from build123d import *

# Parameters (mm, degrees)
SKETCH1_W               = 38.1
SKETCH1_H               = 127
BOSS_EXTRUDE1_DEPTH     = 57.15
SKETCH2_W               = 21.59
SKETCH2_H               = 254
CUT_EXTRUDE1_DEPTH      = 46.99
CUT_EXTRUDE2_DEPTH      = 94.541341128
CUT_EXTRUDE2_DEPTH_BACK = 94.541341128
SKETCH3_R               = 5.08
CUT_EXTRUDE8_START      = -38.1
CUT_EXTRUDE8_DEPTH      = 38.1
SKETCH12_W              = 19.558
SKETCH12_H              = 12.7
CUT_EXTRUDE9_DEPTH      = 140.549828341
SKETCH13_R              = 2.413
CUT_EXTRUDE10_DEPTH     = 80.81826227
F_3_CLEARANCE_HOLE1_D   = 4.5
SKETCH16_R              = 2.2479
CUT_EXTRUDE11_DEPTH     = 93.011478034
CUT_EXTRUDE13_DEPTH     = 6
CUT_EXTRUDE14_DEPTH     = 93.011478034
FILLET3_R               = 2.54


# Read off the part's stored shape, not the designer's step: Cut-Extrude8
with BuildPart() as part:
    # Sketch1 → Boss-Extrude1 (new body)
    with BuildSketch(Plane(origin=(0, 0, 0), x_dir=(1, 0, 0), z_dir=(0, 1, 0))):
        Rectangle(SKETCH1_W, SKETCH1_H)
    extrude(amount=BOSS_EXTRUDE1_DEPTH)

    # Sketch2 → Cut-Extrude1 (cut)
    with BuildSketch(Plane(origin=(0, 57.15, 0), x_dir=(1, 0, 0), z_dir=(0, 1, 0))):
        with Locations((0, -31.75)):
            Rectangle(SKETCH2_W, SKETCH2_H)
    extrude(amount=-CUT_EXTRUDE1_DEPTH, mode=Mode.SUBTRACT)

    # Sketch3 → Cut-Extrude2 (cut, two sides: drawn at the far end of the back side and taken through both)
    with BuildSketch(Plane(origin=(19.05, 0, 0), x_dir=(0, 0, -1), z_dir=(1, 0, 0)).offset(-CUT_EXTRUDE2_DEPTH_BACK)):
        with Locations((-31.75, 29.21)):
            Circle(SKETCH3_R)
        with Locations((31.75, 29.21)):
            Circle(SKETCH3_R)
    extrude(amount=CUT_EXTRUDE2_DEPTH + CUT_EXTRUDE2_DEPTH_BACK, mode=Mode.SUBTRACT)

    # Cut-Extrude8 outline → Cut-Extrude8 (cut)
    with BuildSketch(Plane.ZY.offset(19.05).offset(CUT_EXTRUDE8_START)):
        with BuildLine():
            Line((-63.5, 26.142048402), (-56.964037289, 26.142048402))
            ThreePointArc((-56.964037289, 26.142048402), (-31.750000056, 54.609999908), (-6.535962824, 26.142048402))
            Line((-6.535962824, 26.142048402), (24.774896202, 26.142048402))
            ThreePointArc((24.774896202, 26.142048402), (32.165934032, 36.818639752), (38.349113577, 25.4))
            Line((38.349113577, 25.4), (63.5, 25.4))
            Line((63.5, 25.4), (63.5, 57.15))
            Line((63.5, 57.15), (-63.5, 57.15))
            Line((-63.5, 57.15), (-63.5, 26.142048402))
        make_face()
    extrude(amount=CUT_EXTRUDE8_DEPTH, mode=Mode.SUBTRACT)

    # Sketch12 → Cut-Extrude9 (cut, through all)
    with BuildSketch(Plane.XY.offset(63.5)):
        Rectangle(SKETCH12_W, SKETCH12_H)
    extrude(amount=-CUT_EXTRUDE9_DEPTH, mode=Mode.SUBTRACT)

    # Sketch13 → Cut-Extrude10 (cut, through all)
    with BuildSketch(Plane(origin=(0, 10.16, 0), x_dir=(1, 0, 0), z_dir=(0, 1, 0))):
        with Locations(Location((0, -44.45, 0), (0, 0, 270))):
            Circle(SKETCH13_R)
        with Locations(Location((0, 57.15, 0), (0, 0, 270))):
            Circle(SKETCH13_R)
        with Locations(Location((0, 6.35, 0), (0, 0, 270))):
            Circle(SKETCH13_R)
    extrude(amount=-CUT_EXTRUDE10_DEPTH, mode=Mode.SUBTRACT)

    # 3 Clearance Hole1 (through all)
    with Locations(Plane.ZY.offset(19.05)):
        with Locations((-21.766489637, 45.37568946), (-41.733510476, 13.044310357)):
            Hole(F_3_CLEARANCE_HOLE1_D / 2)

    # Sketch16 → Cut-Extrude11 (cut, through all)
    with BuildSketch(Plane.ZY.offset(19.05)):
        with Locations((-47.200000057, 29.209999908)):
            Circle(SKETCH16_R)
        with Locations((-16.300000057, 29.209999908)):
            Circle(SKETCH16_R)
    extrude(amount=-CUT_EXTRUDE11_DEPTH, mode=Mode.SUBTRACT)

    # Sketch21 → Cut-Extrude13 (cut)
    with BuildSketch(Plane.ZY.offset(19.05)):
        with BuildLine():
            Line((-49.051132759, 36.116215079), (-34.636731482, 39.979832013))
            Line((-34.636731482, 39.979832013), (-28.863268699, 39.979832039))
            Line((-28.863268699, 39.979832039), (-14.448867387, 36.116215233))
            ThreePointArc((-14.448867387, 36.116215233), (-9.150000043, 29.210000101), (-14.448867326, 22.303784921))
            Line((-14.448867326, 22.303784921), (-28.863268603, 18.440167987))
            Line((-28.863268603, 18.440167987), (-34.636731386, 18.440167961))
            Line((-34.636731386, 18.440167961), (-49.051132698, 22.303784767))
            ThreePointArc((-49.051132698, 22.303784767), (-54.350000043, 29.209999899), (-49.051132759, 36.116215079))
        make_face()
    cut_extrude13 = extrude(amount=-CUT_EXTRUDE13_DEPTH, mode=Mode.SUBTRACT)

    # Sketch22 → Cut-Extrude14 (cut, through all)
    with BuildSketch(Plane.ZY.offset(19.05)):
        Polygon((-56.683234461, 34.057042479), (-39.570689377, 39.862220003), (-27.251193914, 54.208414749), (-28.68815775, 55.797566838), (-55.153027555, 53.24322782), (-63.3901932, 32.021075452), align=None)
    extrude(amount=-CUT_EXTRUDE14_DEPTH, mode=Mode.SUBTRACT)

    # Fillet3
    fillet3_edges = [part.edges().sort_by_distance(p)[0] for p in [
        (14.4145, 0, 63.5),
        (-14.4145, 0, -63.5),
        (14.9225, 54.208414749, -27.251193914),
        (-14.9225, 54.208414749, -27.251193914),
        (14.9225, 39.862220003, -39.570689377),
        (-14.9225, 39.862220003, -39.570689377),
        (14.9225, 34.057042479, -56.683234461),
        (-14.9225, 34.057042479, -56.683234461),
        (-14.4145, 0, 63.5),
        (14.4145, 0, -63.5),
        (14.9225, 26.142048402, -6.535962824),
        (-14.9225, 26.142048402, -6.535962824),
        (14.9225, 26.142048402, -56.964037289),
        (-14.9225, 26.142048402, -56.964037289),
        (14.9225, 26.142048402, -63.5),
        (-14.9225, 26.142048402, -63.5),
        (14.9225, 25.4, 63.5),
        (-14.9225, 25.4, 63.5),
        (14.9225, 25.4, 38.349113577),
        (-14.9225, 25.4, 38.349113577),
        (14.9225, 26.142048402, 24.774896202),
        (-14.9225, 26.142048402, 24.774896202),
    ]]
    fillet(fillet3_edges, radius=FILLET3_R)

    # Mirror1: Cut-Extrude13 across plane
    add(cut_extrude13.mirror(Plane(origin=(0, 0, 0), x_dir=(0, 0, 1), z_dir=(1, 0, 0))), mode=Mode.SUBTRACT)


solid = part.part
Here's how the part is built. I have some questions about the finished solid (model axes, mm). A direction names the side the tool comes from. Give positions to 0.01 mm unless a question says otherwise; leave off trailing zeros. Write each loop counter-clockwise with the first axis right and the second up, starting at its lowest first coordinate (ties: lowest second). Pieces come first, ordered by that corner, then holes. Notation, with made-up numbers: (53, 0.25) -> (62, 0.25) arc R17 ccw to (62, 4.25) -> close; hole circle Ø4 at (18, -13.5). An arc over 180 degrees is marked (long way). Use one line per item in the form item = value. Start each with the question number.
1. Imagine slicing it at B-B on y = 16.5. List the corners of the cut face in (x, z) for me (3 decimals).
2. Thinking about a two-plate mould opening in X: for faces 6 (the face through (-13.05, 29, -26)), 7 (the face through (0.725, 8.282, -54.848)), 8 (the face through (-14.865, 30.577, -57.113)), which applies, +X half, -X half, draft (parallel to the pull), parting line (faces both ways), or undercut?
3. Imagine slicing it at D-D on z = 45. List the corners of the cut face in (x, y) for me (3 decimals).
4. Imagine slicing it at A-A on z = 31.75. List the corners of the cut face in (x, y) for me (3 decimals), plus the area to 3 significant figures.
5. Imagine slicing it at C-C on x = 0. List the corners of the cut face in (y, z) for me, plus the area to 3 significant figures.
6. Will these pins go through, and if not, where does the flat tip stop? pin 1 Ø1 at (x, z) = (-4.5, -25) entering from -Y; pin 2 Ø5 at (x, z) = (-10, -48.5) entering from +Y; pin 3 Ø5 at (y, z) = (29.21, -47.2) entering from +X.
7. If I drill on L1, parallel to Z at x = -12, y = 29; L2, parallel to X at y = 17.5, z = -2 (3 decimals), over which ranges is the centre line in solid material (lowest first)?
8. On a 3-axis mill with a long thin cutter (end or side, diameter ignored), from which of +Z, -Z, +X, -X, +Y, -Y can I reach the whole of each face in a straight line? I mean faces 1 (the face through (-16.092, 38.021, -41.945)), 2 (the face through (16.09, 29.08, -54.35)), 3 (the face through (15, 25.4, 51)), 4 (the face through (11.91, 27.26, -36.44)), 5 (the face through (-10.795, 23, -13)). Say none if no direction works.
Entries:
q1.outline = (-19.05, -63.5) -> (-10.795, -63.5) -> (-10.795, 63.5) -> (-19.05, 63.5) -> close; (10.795, -63.5) -> (19.05, -63.5) -> (19.05, 63.5) -> (10.795, 63.5) -> close
q2.face_6 = -X half
q2.face_7 = undercut
q2.face_8 = draft
q3.outline = (-19.05, 0) -> (-9.779, 0) -> (-9.779, 6.35) -> (-2.349, 6.35) -> (-2.349, 10.16) -> (-10.795, 10.16) -> (-10.795, 25.4) -> (-19.05, 25.4) -> close; (2.349, 6.35) -> (9.779, 6.35) -> (9.779, 0) -> (19.05, 0) -> (19.05, 25.4) -> (10.795, 25.4) -> (10.795, 10.16) -> (2.349, 10.16) -> close
q4.outline = (-19.05, 0) -> (-9.779, 0) -> (-9.779, 6.35) -> (9.779, 6.35) -> (9.779, 0) -> (19.05, 0) -> (19.05, 24.13) -> (10.795, 24.13) -> (10.795, 10.16) -> (-10.795, 10.16) -> (-10.795, 24.13) -> (-19.05, 24.13) -> close; (-19.05, 34.29) -> (-10.795, 34.29) -> (-10.795, 36.83) -> (-19.05, 36.83) -> close; (10.795, 34.29) -> (19.05, 34.29) -> (19.05, 36.83) -> (10.795, 36.83) -> close
q4.area = 535 mm²
q5.outline = (6.35, -63.5) -> (10.16, -63.5) -> (10.16, -59.56) -> (6.35, -59.56) -> close; (6.35, -54.74) -> (10.16, -54.74) -> (10.16, -8.76) -> (6.35, -8.76) -> close; (6.35, -3.94) -> (10.16, -3.94) -> (10.16, 42.04) -> (6.35, 42.04) -> close; (6.35, 46.86) -> (10.16, 46.86) -> (10.16, 63.5) -> (6.35, 63.5) -> close
q5.area = 429 mm²
q6.pin_1 = 6.35
q6.pin_2 = 37.64
q6.pin_3 = 13.05
q7.L1 = -57.15 to -49.44, -44.96 to -36.83, -26.67 to -18.54, -14.06 to -6.35, 24.13 to 26.67, 36.83 to 39.37
q7.L2 = -19.05 to -10.795, 10.795 to 19.05
q8.face_1 = -X
q8.face_2 = +X
q8.face_3 = +Z, +X, -X, +Y
q8.face_4 = +X, -X
q8.face_5 = +Z, -Z, +Y
